from build123d import *

# Parameters (mm, degrees)
SKETCH1_W           = 60
SKETCH1_H           = 100
BOSS_EXTRUDE1_DEPTH = 100
SKETCH2_W           = 50
SKETCH2_H           = 100
CUT_EXTRUDE1_DEPTH  = 40
SKETCH3_W           = 5
SKETCH3_H           = 100
BOSS_EXTRUDE2_DEPTH = 30
SKETCH4_W           = 100
SKETCH4_H           = 10
BOSS_EXTRUDE3_DEPTH = 10
SKETCH5_W           = 60
SKETCH5_H           = 80
BOSS_EXTRUDE4_DEPTH = 350
SKETCH6_W           = 50
SKETCH6_H           = 100
CUT_EXTRUDE2_DEPTH  = 50
SKETCH7_R           = 10
CUT_EXTRUDE3_DEPTH  = 80
SKETCH8_W           = 50
SKETCH8_H           = 35
CUT_EXTRUDE4_DEPTH  = 350
SKETCH9_W           = 5
SKETCH9_H           = 30
CUT_EXTRUDE5_DEPTH  = 350


with BuildPart() as part:
    # Sketch1 → Boss-Extrude1 (new body)
    with BuildSketch(Plane(origin=(0, 0, 0), x_dir=(1, 0, 0), z_dir=(0, 1, 0))):
        with Locations((-100.731707317, 49.268292683)):
            Rectangle(SKETCH1_W, SKETCH1_H)
    extrude(amount=BOSS_EXTRUDE1_DEPTH)

    # Sketch2 → Cut-Extrude1 (cut)
    with BuildSketch(Plane(origin=(0, 100, 0), x_dir=(1, 0, 0), z_dir=(0, 1, 0))):
        with Locations((-100.731707317, 49.268292683)):
            Rectangle(SKETCH2_W, SKETCH2_H)
    extrude(amount=-CUT_EXTRUDE1_DEPTH, mode=Mode.SUBTRACT)

    # Sketch3 → Boss-Extrude2 (add)
    with BuildSketch(Plane(origin=(0, 100, 0), x_dir=(1, 0, 0), z_dir=(0, 1, 0))):
        with Locations((-73.231707317, 49.268292683)):
            Rectangle(SKETCH3_W, SKETCH3_H)
    extrude(amount=BOSS_EXTRUDE2_DEPTH)

    # Sketch4 → Boss-Extrude3 (add)
    with BuildSketch(Plane.ZY.offset(75.731707317)):
        with Locations((-49.268292683, 125)):
            Rectangle(SKETCH4_W, SKETCH4_H)
    extrude(amount=BOSS_EXTRUDE3_DEPTH)

    # Sketch5 → Boss-Extrude4 (add)
    with BuildSketch(Plane(origin=(0, 0, 0), x_dir=(-1, 0, 0), z_dir=(0, -1, 0))):
        with Locations((100.731707317, 49.268292683)):
            Rectangle(SKETCH5_W, SKETCH5_H)
    extrude(amount=BOSS_EXTRUDE4_DEPTH)

    # Sketch6 → Cut-Extrude2 (cut)
    with BuildSketch(Plane(origin=(0, 60, 0), x_dir=(1, 0, 0), z_dir=(0, 1, 0))):
        with Locations((-100.731707317, 49.268292683)):
            Rectangle(SKETCH6_W, SKETCH6_H)
    extrude(amount=-CUT_EXTRUDE2_DEPTH, mode=Mode.SUBTRACT)

    # Sketch7 → Cut-Extrude3 (cut)
    with BuildSketch(Plane.ZY.offset(130.731707317)):
        with Locations((-49.268292683, 35)):
            Circle(SKETCH7_R)
    extrude(amount=-CUT_EXTRUDE3_DEPTH, mode=Mode.SUBTRACT)

    # Sketch8 → Cut-Extrude4 (cut)
    with BuildSketch(Plane(origin=(0, -350, 0), x_dir=(-1, 0, 0), z_dir=(0, -1, 0))):
        with Locations((100.731707317, 26.768292683)):
            Rectangle(SKETCH8_W, SKETCH8_H)
        with Locations((100.731707317, 71.768292683)):
            Rectangle(SKETCH8_W, SKETCH8_H)
    extrude(amount=-CUT_EXTRUDE4_DEPTH, mode=Mode.SUBTRACT)

    # Sketch9 → Cut-Extrude5 (cut)
    with BuildSketch(Plane(origin=(0, -350, 0), x_dir=(-1, 0, 0), z_dir=(0, -1, 0))):
        with Locations((128.231707317, 74.268292683)):
            Rectangle(SKETCH9_W, SKETCH9_H)
        with Locations((128.231707317, 24.268292683)):
            Rectangle(SKETCH9_W, SKETCH9_H)
    extrude(amount=-CUT_EXTRUDE5_DEPTH, mode=Mode.SUBTRACT)


solid = part.part
Design review of the part built by this model. Coordinates are the model's own, in mm. A direction names the side the tool comes from. Give positions to 0.01 mm unless a question says otherwise; leave off trailing zeros. Loops run counter-clockwise (first coordinate to the right, second up) from the corner with the lowest first, then second, coordinate; pieces in that order, holes last. Notation, with made-up numbers: M 67.25,7.5 L 116.25,7.5 A24 cw 116.25,17.5 Z; hole C -40,-33.75 d6. An arc over 180 degrees is marked long. Write item = value, one per line.
Q1. Insertion check: pin 1 (2.5 mm diameter, centred on x = -73.5, y = -203, fed in from -Z); pin 2 (8 mm diameter, centred on y = 126.5, z = -24.5, fed in from -X); pin 3 (2.5 mm diameter, centred on x = -127, y = -247, fed in from -Z). Each pin has a flat end and moves straight along its axis. Give the tip position at first contact, or say it passes through.
Output values:
pin_1 = -89.27
pin_2 = -85.73
pin_3 = -59.27
Q2. We need section D-D (x = -105). Give the boundary of the cut face in (y, z), plus the area to 3 significant figures.
Output values:
outline = M -350,-54.27 L 0,-54.27 L 0,-99.27 L 10,-99.27 L 10,0.73 L 0,0.73 L 0,-44.27 L -350,-44.27 Z
area = 4,500 mm^2
Q3. For faces 5 (the flat face through (-75.732, 64, -49)), 6 (the flat face through (-100, -177, -44.268)), 7 (the flat face through (-85.732, 125, -50)), 8 (the flat face through (-100, -177, -54.268)), 9 (the flat face through (-81, 120, -50)), list the 3-axis set-ups (+Z, -Z, +X, -X, +Y, -Y) from which the entire face can be reached by the end or side of a thin tool; tool diameter is ignored.
Output values:
face_5 = +Z, -Z
face_6 = +Z, -Y
face_7 = +Z, -Z, -X, +Y
face_8 = -Z, -Y
face_9 = +Z, -Z, -X
Q4. Draft analysis for pull direction Y (two halves, no side actions). For faces 1 (the flat face through (-78, 130, -50)), 2 (the cylindrical face through (-128.27, 25.24, -51.44)), 3 (the flat face through (-92, -350, -49)), 4 (the flat face through (-75.732, -177, -72)), state which applies: +Y half, -Y half, draft (parallel to the pull), parting line (faces both ways), or undercut.
Output values:
face_1 = +Y half
face_2 = undercut
face_3 = -Y half
face_4 = draft
Q5. We need section C-C (z = -75). Give the boundary of the cut face in (x, y), plus the area to 3 significant figures.
Output values:
outline = M -130.73,0 L -75.73,0 L -75.73,-350 L -70.73,-350 L -70.73,130 L -85.73,130 L -85.73,120 L -75.73,120 L -75.73,10 L -125.73,10 L -125.73,100 L -130.73,100 Z
area = 3,500 mm^2
Q6. To check wall thickness, follow line 1 (X direction, y = 67, z = -14); line 2 (Y direction, x = -84, z = -85.5); line 3 (Y direction, x = -114.5, z = -74). State the ranges of each line that lie inside material, in increasing order. Write a range as [from, to].
Output values:
line_1 = [-130.73, -125.73], [-75.73, -70.73]
line_2 = [0, 10], [120, 130]
line_3 = [0, 10]
Q7. We need section A-A (y = 35). Give the boundary of the cut face in (x, z), plus the area to 3 significant figures.
Output values:
outline = M -130.73,-99.27 L -125.73,-99.27 L -125.73,-59.27 L -130.73,-59.27 Z; M -130.73,-39.27 L -125.73,-39.27 L -125.73,0.73 L -130.73,0.73 Z; M -75.73,-99.27 L -70.73,-99.27 L -70.73,-59.27 L -75.73,-59.27 Z; M -75.73,-39.27 L -70.73,-39.27 L -70.73,0.73 L -75.73,0.73 Z
area = 800 mm^2
Q8. We need section B-B (x = -81.5). Give the boundary of the cut face in (y, z).
Output values:
outline = M -350,-54.27 L 0,-54.27 L 0,-99.27 L 10,-99.27 L 10,0.73 L 0,0.73 L 0,-44.27 L -350,-44.27 Z; M 120,-99.27 L 130,-99.27 L 130,0.73 L 120,0.73 Z
